from build123d import *

# Parameters (mm, degrees)
EXTRUDE_THIN1_DEPTH = 381
FILLET1_R           = 1.27


with BuildPart() as part:
    # Sketch1 → Extrude-Thin1 (new body)
    with BuildSketch(Plane.XY):
        with BuildLine():
            Line((0, 0), (-3.578277876, 0))
            ThreePointArc((-3.578277876, 0), (-11.355407809, 2.659768429), (-15.875, 9.525))
            Line((-15.875, 9.525), (-19.05, 9.525))
            Line((-19.05, 9.525), (-19.05, 34.925))
            Line((-19.05, 34.925), (-15.875, 34.925))
            Line((-15.875, 34.925), (-15.875, 38.1))
            Line((-15.875, 38.1), (0, 38.1))
            Line((0, 38.1), (0, 36.83))
            Line((0, 36.83), (-14.605, 36.83))
            Line((-14.605, 36.83), (-14.605, 33.655))
            Line((-14.605, 33.655), (-17.78, 33.655))
            Line((-17.78, 33.655), (-17.78, 10.795))
            Line((-17.78, 10.795), (-14.848409863, 10.795))
            ThreePointArc((-14.848409863, 10.795), (-10.95631115, 3.970193301), (-3.578277876, 1.27))
            Line((-3.578277876, 1.27), (0, 1.27))
            Line((0, 1.27), (0, 0))
        make_face()
    extrude(amount=-EXTRUDE_THIN1_DEPTH)

    # Fillet1
    fillet1_edges = [part.edges().sort_by_distance(p)[0] for p in [
        (-14.605, 33.655, -190.5),
        (-14.848409863, 10.795, -190.5),
        (-19.05, 9.525, -190.5),
        (-19.05, 34.925, -190.5),
        (-15.875, 38.1, -190.5),
    ]]
    fillet(fillet1_edges, radius=FILLET1_R)


solid = part.part
Verification items for the finished model (mm, model axes). A direction names the side the tool comes from. Give positions to 0.01 mm unless a question says otherwise; leave off trailing zeros. Order: outer loops, then holes, each group sorted by start corner. A loop starts at its lowest first (then second) coordinate and runs counter-clockwise, first axis right, second up. Notation, with made-up numbers: (42, -14.75) -> (68, -14.75) arc R21 ccw to (68, 5.25) -> close; hole circle Ø10 at (50, 79.5). An arc over 180 degrees is marked (long way). Answer as CSV lines item,"result".
Q1. Sectioned sample at C-C on y = 4.5. Record the cut outline in (x, z).
Solutions:
outline,"(-13.28, -381) -> (-11.54, -381) -> (-11.54, 0) -> (-13.28, 0) -> close"
Q2. Sectioned sample at B-B on y = 28.5. Record the cut outline in (x, z).
Solutions:
outline,"(-19.05, -381) -> (-17.78, -381) -> (-17.78, 0) -> (-19.05, 0) -> close"
Q3. Scan lines: probe 1 along Y at (x, z) = (-2.5, -254.5); probe 2 along Y at (x, z) = (-16.5, -193) (3 decimals); probe 3 along X at (y, z) = (12, -203). Record each from-to range of solid material in increasing order.
Solutions:
probe 1,"y = 0 to 1.27, 36.83 to 38.1"
probe 2,"y = 9.525 to 10.795, 33.655 to 34.925"
probe 3,"x = -19.05 to -17.78"
Q4. Depth check by flat-ended pin: pin 1 (7.5 mm diameter, centred on x = -10.5, z = -96.5, fed in from -Y); pin 2 (1.5 mm diameter, centred on y = 36, z = -123.5, fed in from +X) (3 decimals); pin 3 (0.6 mm diameter, centred on y = 36, z = -256, fed in from -X) (3 decimals). Enter the tip coordinate at first touch or a pass-through.
Solutions:
pin 1,"stops at y = 0.4"
pin 2,"stops at x = -14.605"
pin 3,"stops at x = -15.875"
Q5. Access from +Z, -Z, +X, -X, +Y, -Y to the whole of each face (thin tool, end or side, straight path). Record for faces 1 (the cylindrical face through (-11.262, 2.588, -187.833)), 2 (the cylindrical face through (-10.66, 3.73, -187.83)).
Solutions:
face 1,"+Z, -Z, -X, -Y"
face 2,"+Z, -Z, +X"
Q6. Release check for a two-part mould opening along Y. For faces 3 (the flat face through (-7, 36.83, -188)), 4 (the flat face through (-19.05, 22, -188)), 5 (the flat face through (-7, 38.1, -188)), 6 (the flat face through (-17.78, 22, -188)) record: +Y half, -Y half, draft (parallel to the pull), parting line (faces both ways), or undercut.
Solutions:
face 3,"undercut"
face 4,"draft"
face 5,"+Y half"
face 6,"undercut"
